from build123d import *

# Parameters (mm, degrees)
F0_R     = 43.5
F0_R_2   = 38.5
F1_DEPTH = 10
F2_R     = 40.5
F2_R_2   = 38.5
F3_DEPTH = 90
F4_R     = 38.5
F5_DEPTH = 2
F6_R     = 1


with BuildPart() as f1:
    # F0 (on Top) → F1 (new body)
    with BuildSketch(Plane.XY):
        Circle(F0_R)
        Circle(F0_R_2, mode=Mode.SUBTRACT)
    extrude(amount=F1_DEPTH)

    # F2 (on face) → F3 (join)
    with BuildSketch(Plane.XY.offset(10)):
        Circle(F2_R)
        Circle(F2_R_2, mode=Mode.SUBTRACT)
    extrude(amount=F3_DEPTH)

    # F4 (on face) → F5 (join)
    with BuildSketch(Plane.XY.offset(100)):
        Circle(F4_R)
    extrude(amount=-F5_DEPTH)

    # F6
    f6_edges = [f1.edges().sort_by_distance(p)[0] for p in [
        (-43.5, 0, 0),
        (-38.5, 0, 0),
        (-40.5, 0, 100),
        (-38.5, 0, 98),
    ]]
    fillet(f6_edges, radius=F6_R)


solid = f1.part
Design review of the part built by this model. Coordinates are the model's own, in mm. Round coordinates to 2 decimals unless told otherwise and drop trailing zeros. Write each loop counter-clockwise with the first axis right and the second up, starting at its lowest first coordinate (ties: lowest second). Pieces come first, ordered by that corner, then holes.
Item 1: Consider section A-A on x = 0. Give the boundary of the cut face in (y, z).
Item 2: Draft analysis for pull direction X (two halves, no side actions). For faces 1 (the flat face through (-1, 1, 98)), 2 (the cylindrical face through (21.77, 34.15, 53.88)), 3 (the flat face through (29, -29, 10)), 4 (the cylindrical face through (-30.55, -23.43, 48.33)), state which applies: released by +X, released by -X, zero draft, split by the parting line, or undercut.
Item 3: Consider section B-B on z = 52.5. Give the boundary of the cut face in (x, y), and give its area (3 significant figures).
Item 4: Wall thickness on L1, parallel to Y at x = 0, z = 32; L2, parallel to X at y = 1, z = 74.5; L3, parallel to X at y = 12, z = 22: over which ranges is each line inside the solid? List them lowest first.
Item 5: For pin 1 Ø8 at (y, z) = (30, 39) entering from +X; pin 2 Ø10 at (y, z) = (-10.5, 59.5) entering from -X; pin 3 Ø6 at (y, z) = (19, 48) entering from -X, all flat-tipped, find the tip position at first contact; note any pin that passes through.
Check values:
1. outline: (-43.5, 1) arc R1 ccw to (-42.5, 0) - (-39.5, 0) arc R1 ccw to (-38.5, 1) - (-38.5, 97) arc R1 cw to (-37.5, 98) - (37.5, 98) arc R1 cw to (38.5, 97) - (38.5, 1) arc R1 ccw to (39.5, 0) - (42.5, 0) arc R1 ccw to (43.5, 1) - (43.5, 10) - (40.5, 10) - (40.5, 99) arc R1 ccw to (39.5, 100) - (-39.5, 100) arc R1 ccw to (-40.5, 99) - (-40.5, 10) - (-43.5, 10) - close
2. face 1: undercut
2. face 2: split by the parting line
2. face 3: zero draft
2. face 4: undercut
3. outline: circle Ø81 at (0, 0); hole circle Ø77 at (0, 0)
3. area: 496 mm2
4. L1: y = -40.5 to -38.5, 38.5 to 40.5
4. L2: x = -40.49 to -38.49, 38.49 to 40.49
4. L3: x = -38.68 to -36.58, 36.58 to 38.68
5. pin 1: stops at x = 31.05
5. pin 2: stops at x = -40.12
5. pin 3: stops at x = -37.21
